from build123d import *

# Parameters (mm, degrees)
SKETCH1_W           = 135
SKETCH1_H           = 35
BOSS_EXTRUDE1_DEPTH = 10
FILLET1_R           = 20
SKETCH3_R           = 12.75
CUT_EXTRUDE1_DEPTH  = 2
SKETCH4_R           = 11.5
CUT_EXTRUDE2_DEPTH  = 6
CUT_EXTRUDE3_REACH  = 93.483
SKETCH5_R           = 1.75
SKETCH6_R           = 3.1
CUT_EXTRUDE4_DEPTH  = 4
FILLET2_R           = 15


with BuildPart() as part:
    # Sketch1 → Boss-Extrude1 (new body)
    with BuildSketch(Plane(origin=(0, 0, 0), x_dir=(1, 0, 0), z_dir=(0, 1, 0))):
        with Locations((19.749798241, -8.123070146)):
            Rectangle(SKETCH1_W, SKETCH1_H)
    extrude(amount=BOSS_EXTRUDE1_DEPTH)

    # Fillet1
    fillet1_edges = [part.edges().sort_by_distance(p)[0] for p in [
        (87.249798241, 5, 25.623070146),
        (-47.750201759, 5, 25.623070146),
    ]]
    fillet(fillet1_edges, radius=FILLET1_R)

    # Sketch3 → Cut-Extrude1 (cut)
    with BuildSketch(Plane(origin=(0, 10, 0), x_dir=(1, 0, 0), z_dir=(0, 1, 0))):
        with Locations(Location((-27.750201759, -6.88629089, 0), (0, 0, 270))):
            Circle(SKETCH3_R)
        with Locations(Location((67.249798241, -6.88629089, 0), (0, 0, 90))):
            Circle(SKETCH3_R)
    extrude(amount=-CUT_EXTRUDE1_DEPTH, mode=Mode.SUBTRACT)

    # Sketch4 → Cut-Extrude2 (cut)
    with BuildSketch(Plane(origin=(0, 8, 0), x_dir=(1, 0, 0), z_dir=(0, 1, 0))):
        with Locations(Location((-27.750201759, -6.88629089, 0), (0, 0, 270))):
            Circle(SKETCH4_R)
        with Locations(Location((67.249798241, -6.88629089, 0), (0, 0, 90))):
            Circle(SKETCH4_R)
    extrude(amount=-CUT_EXTRUDE2_DEPTH, mode=Mode.SUBTRACT)

    # Sketch5 → Cut-Extrude3 (cut, up to next)
    with BuildSketch(Plane(origin=(0, 10, 0), x_dir=(1, 0, 0), z_dir=(0, 1, 0)), mode=Mode.PRIVATE) as cut_extrude3_sk1:
        with Locations(Location((19.749798241, -0.623070146, 0), (0, 0, 270))):
            Circle(SKETCH5_R)
    cut_extrude3_tool1 = extrude(cut_extrude3_sk1.sketch, amount=-CUT_EXTRUDE3_REACH, mode=Mode.PRIVATE) & part.part
    # Sketch5 → Cut-Extrude3 (cut, up to next)
    with BuildSketch(Plane(origin=(0, 10, 0), x_dir=(1, 0, 0), z_dir=(0, 1, 0)), mode=Mode.PRIVATE) as cut_extrude3_sk2:
        with Locations(Location((19.749798241, -15.623070146, 0), (0, 0, 270))):
            Circle(SKETCH5_R)
    cut_extrude3_tool2 = extrude(cut_extrude3_sk2.sketch, amount=-CUT_EXTRUDE3_REACH, mode=Mode.PRIVATE) & part.part
    add(cut_extrude3_tool1.solids().sort_by_distance((19.749798, 10, 0.62307))[0], mode=Mode.SUBTRACT)
    add(cut_extrude3_tool2.solids().sort_by_distance((19.749798, 10, 15.62307))[0], mode=Mode.SUBTRACT)

    # Sketch6 → Cut-Extrude4 (cut)
    with BuildSketch(Plane.XZ):
        with Locations(Location((19.749798241, 15.623070146, 0), (0, 0, 270))):
            Circle(SKETCH6_R)
        with Locations(Location((19.749798241, 0.623070146, 0), (0, 0, 270))):
            Circle(SKETCH6_R)
    extrude(amount=-CUT_EXTRUDE4_DEPTH, mode=Mode.SUBTRACT)

    # Fillet2
    fillet2_edges = [part.edges().sort_by_distance(p)[0] for p in [
        (-47.750201759, 5, -9.376929854),
        (87.249798241, 5, -9.376929854),
    ]]
    fillet(fillet2_edges, radius=FILLET2_R - 0.0001)  # a hair under: the kernel refuses the full size


solid = part.part
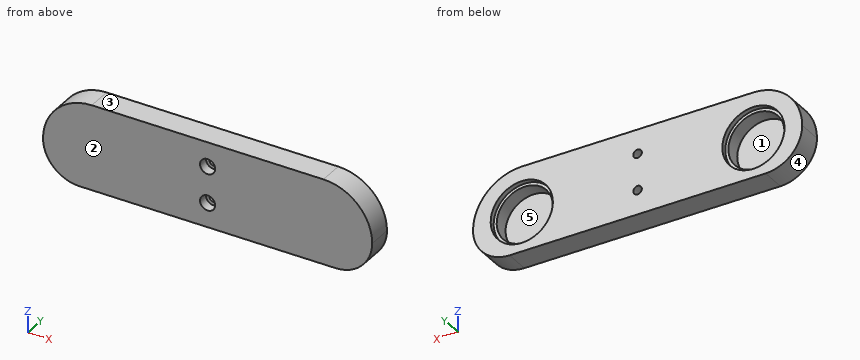
Input: part model. Units: mm. Frame: model coordinates. Face numbers are marked on the shaded views. A direction names the side the tool comes from. Give positions to 0.01 mm unless a question says otherwise; leave off trailing zeros. Write each loop counter-clockwise with the first axis right and the second up, starting at its lowest first coordinate (ties: lowest second). Pieces come first, ordered by that corner, then holes. Notation, with made-up numbers: M -1.75,32 L 26.25,32 A22 cw 26.25,71 Z; hole C -10.75,18.5 d8. An arc over 180 degrees is marked long. Use one line per item in the form item = value.
1. Ray query, L1, parallel to X at y = 5, z = 9; L2, parallel to X at y = 9, z = 8; L3, parallel to X at y = 7.5, z = 17. Return the intervals inside material, ascending.
Outcome:
L1 = -47.46 to -39.05, -16.45 to 55.95, 78.55 to 86.96
L2 = -47.61 to -40.45, -15.05 to 54.55, 79.95 to 87.11
L3 = -44.2 to -33.22, -22.28 to 18.67, 20.83 to 61.78, 72.72 to 83.7
2. Cut plane A-A on z = 16. Return loops of the section in (x, y), and give its area (3 significant figures).
Outcome:
outline = M -44.85,0 L 16.67,0 L 16.67,4 L 18.04,4 L 18.04,10 L -18.83,10 L -18.83,8 L -20.74,8 L -20.74,2 L -34.76,2 L -34.76,8 L -36.67,8 L -36.67,10 L -44.85,10 Z; M 21.46,4 L 22.83,4 L 22.83,0 L 84.35,0 L 84.35,10 L 76.17,10 L 76.17,8 L 74.26,8 L 74.26,2 L 60.24,2 L 60.24,8 L 58.33,8 L 58.33,10 L 21.46,10 Z
area = 1,010 mm²
3. First-contact query: P1, Ø3, axis at x = 19.75, z = 0.62, coming from the +Y side; P2, Ø3, axis at x = 19, z = 2, coming from the -Y side; P3, Ø3, axis at y = 5.5, z = -5.5, coming from the -X side; P4, Ø1.5, axis at y = 3, z = 13.5, coming from the +X side. Flat tips, straight axial feed; report the tip coordinate or a pass-through.
Outcome:
P1 = through
P2 = 4
P3 = -44.26
P4 = 85.94
4. Cut plane C-C on x = 77.5. Return loops of the section in (y, z), and give its area (3 significant figures).
Outcome:
outline = M 0,-8.43 L 10,-8.43 L 10,-0.7 L 8,-0.7 L 8,1.67 L 2,1.67 L 2,12.1 L 8,12.1 L 8,14.47 L 10,14.47 L 10,22.8 L 0,22.8 Z
area = 219 mm²
5. Cut plane D-D on z = 11. Return loops of the section in (x, y), and give its area (3 significant figures).
Outcome:
outline = M -47.01,0 L 86.51,0 L 86.51,10 L 79.32,10 L 79.32,8 L 77.99,8 L 77.99,2 L 56.51,2 L 56.51,8 L 55.18,8 L 55.18,10 L -15.68,10 L -15.68,8 L -17.01,8 L -17.01,2 L -38.49,2 L -38.49,8 L -39.82,8 L -39.82,10 L -47.01,10 Z
area = 981 mm²
6. Cut plane B-B on y = 5.5. State how many separate pieces and enclosed holes the cut face has, and give its area (3 significant figures).
Outcome:
separate_pieces = 1
enclosed_holes = 4
area = 3,610 mm²
7. Mould query, pull axis X, two halves, no side actions, for the marked faces 3, 4 and 5. Classes: released by +X, released by -X, zero draft, split by the parting line, or undercut.
Outcome:
face_3 = zero draft
face_4 = released by -X
face_5 = undercut
8. Reachability of the marked faces 1 and 2 from +Z, -Z, +X, -X, +Y, -Y: full face, straight path, thin tool, end or side. Return the list, or none.
Outcome:
face_1 = +Y
face_2 = +Z, -Z, +X, -X, -Y
